```python
from build123d import *


with BuildPart() as part:
    # Sketch1 → Revolve1 (revolve)
    with BuildSketch(Plane.XY):
        with BuildLine():
            Line((9.207453271, 10), (9.207453271, 14))
            Line((9.207453271, 14), (7.207453271, 14))
            ThreePointArc((7.207453271, 14), (5.086132927, 14.878679656), (4.207453271, 17))
            Line((4.207453271, 17), (4.207453271, 25))
            Line((4.207453271, 25), (-11.792546729, 25))
            Line((-11.792546729, 25), (-11.792546729, 27))
            Line((-11.792546729, 27), (-13.792546729, 27))
            Line((-13.792546729, 27), (-13.792546729, 20))
            Line((-13.792546729, 20), (-0.792546729, 20))
            Line((-0.792546729, 20), (-0.792546729, 10))
            Line((-0.792546729, 10), (9.207453271, 10))
        make_face()
    revolve(axis=Axis((9.207453271, 0, 0), (-1, 0, 0)))


solid = part.part
```
CAD build for the part. Positions are in the model's coordinates, mm. A direction names the side the tool comes from. Give positions to 0.01 mm unless a question says otherwise; leave off trailing zeros. Loops run counter-clockwise (first coordinate to the right, second up) from the corner with the lowest first, then second, coordinate; pieces in that order, holes last. Notation, with made-up numbers: (14.25, -4) -> (57.25, -4) arc R9 ccw to (57.25, 11) -> close; hole circle Ø10 at (16.25, 73). An arc over 180 degrees is marked (long way). Use a Markdown table: item, result.
1. Which spindle directions (+Z, -Z, +X, -X, +Y, -Y) get a long thin tool onto all of the face, cutting with end or side? Do faces 1 (the flat face through (-13.793, -18, 10)), 2 (the cylindrical face through (-7.202, -4.336, 19.524)), 3 (the flat face through (-11.793, -24, 8)). Say none if no direction does.
Check result:
| item | result |
|---|---|
| face 1 | +Z, -Z, -X, +Y, -Y |
| face 2 | -X |
| face 3 | +X |
2. Wall check: L1, parallel to Y at x = 2.75, z = 0; L2, parallel to Y at x = -6, z = 0; L3, parallel to X at y = 10, z = -9.5. Give the ranges that are in metal, low to high. Write a range as [from, to].
Check result:
| item | result |
|---|---|
| L1 | y = [-25, -10], [10, 25] |
| L2 | y = [-25, -20], [20, 25] |
| L3 | x = [-0.79, 9.21] |
3. Slice it at C-C (x = -5.25). List the corners of the cut face in (y, z).
Check result:
| item | result |
|---|---|
| outline | circle Ø50 at (0, 0); hole circle Ø40 at (0, 0) |
4. Flat gauge pins, fed straight in: pin 1 (4 mm diameter, centred on x = -7, z = 2, fed in from +Y); pin 2 (2 mm diameter, centred on x = -7, z = 10, fed in from -Y); pin 3 (1.5 mm diameter, centred on x = -1, z = -10, fed in from -Y). Where does each tip first touch, or does it go through?
Check result:
| item | result |
|---|---|
| pin 1 | stops at y = 25 |
| pin 2 | stops at y = -23.32 |
| pin 3 | stops at y = -23.23 |
5. Mould opens along Z. For faces 4 (the cylindrical face through (8.193, 12.932, 5.362)), 5 (the flat face through (-0.793, -5, -9)), 6 (the flat face through (4.207, 5.9, 16.3)) say: pulls with the +Z half, pulls with the -Z half, needs draft (parallel to the pull), parting line crosses it, or undercut.
Check result:
| item | result |
|---|---|
| face 4 | parting line crosses it |
| face 5 | undercut |
| face 6 | needs draft |
6. Slice it at D-D (z = 22). List the corners of the cut face in (x, y).
Check result:
| item | result |
|---|---|
| outline | (-13.79, -15.65) -> (-11.79, -15.65) -> (-11.79, -11.87) -> (4.21, -11.87) -> (4.21, 11.87) -> (-11.79, 11.87) -> (-11.79, 15.65) -> (-13.79, 15.65) -> close |
7. Slice it at A-A (y = 0). List the corners of the cut face in (x, z), plus the area to 3 significant figures.
Check result:
| item | result |
|---|---|
| outline | (-13.79, -27) -> (-11.79, -27) -> (-11.79, -25) -> (4.21, -25) -> (4.21, -17) arc R3 cw to (7.21, -14) -> (9.21, -14) -> (9.21, -10) -> (-0.79, -10) -> (-0.79, -20) -> (-13.79, -20) -> close; (-13.79, 20) -> (-0.79, 20) -> (-0.79, 10) -> (9.21, 10) -> (9.21, 14) -> (7.21, 14) arc R3 cw to (4.21, 17) -> (4.21, 25) -> (-11.79, 25) -> (-11.79, 27) -> (-13.79, 27) -> close |
| area | 332 mm^2 |
